```python
from build123d import *

# Parameters (mm, degrees)
ESQUISSE1_R             = 1.75
BOSS_EXTRU_1_DEPTH      = 2
ESQUISSE2_R             = 3
ESQUISSE2_R_2           = 1.5621
ESQUISSE2_R_3           = 1.315256363
BOSS_EXTRU_2_DEPTH      = 4
ENL_V_START             = -4
ESQUISSE4_R             = 1.5621
ESQUISSE4_R_2           = 1.315256363
ENL_V_MAT_EXTRU_1_DEPTH = 4


with BuildPart() as part:
    # Esquisse1 → Boss.-Extru.1 (new body)
    with BuildSketch(Plane(origin=(0, 0, 0), x_dir=(1, 0, 0), z_dir=(0, 1, 0))):
        with BuildLine():
            Line((80, 50.039706632), (74.039706632, 50.039706632))
            ThreePointArc((74.039706632, 50.039706632), (70.476095897, 48.563610735), (69, 45))
            ThreePointArc((69, 45), (65.778174593, 37.221825407), (58, 34))
            Line((58, 34), (-58, 34))
            ThreePointArc((-58, 34), (-65.778174593, 37.221825407), (-69, 45))
            ThreePointArc((-69, 45), (-70.476095897, 48.563610735), (-74.039706632, 50.039706632))
            Line((-74.039706632, 50.039706632), (-80, 50.039706632))
            ThreePointArc((-80, 50.039706632), (-83.563610735, 48.563610735), (-85.039706632, 45))
            Line((-85.039706632, 45), (-85.039706632, -45))
            ThreePointArc((-85.039706632, -45), (-83.563610735, -48.563610735), (-80, -50.039706632))
            Line((-80, -50.039706632), (-74.039706632, -50.039706632))
            ThreePointArc((-74.039706632, -50.039706632), (-70.476095897, -48.563610735), (-69, -45))
            ThreePointArc((-69, -45), (-65.778174593, -37.221825407), (-58, -34))
            Line((-58, -34), (58, -34))
            ThreePointArc((58, -34), (65.778174593, -37.221825407), (69, -45))
            ThreePointArc((69, -45), (70.476095897, -48.563610735), (74.039706632, -50.039706632))
            Line((74.039706632, -50.039706632), (80, -50.039706632))
            ThreePointArc((80, -50.039706632), (83.563610735, -48.563610735), (85.039706632, -45))
            Line((85.039706632, -45), (85.039706632, 45))
            ThreePointArc((85.039706632, 45), (83.563610735, 48.563610735), (80, 50.039706632))
        make_face()
        with Locations(Location((-80, -45, 0), (0, 0, 270))):
            Circle(ESQUISSE1_R, mode=Mode.SUBTRACT)
        with Locations(Location((-80, 45, 0), (0, 0, 270))):
            Circle(ESQUISSE1_R, mode=Mode.SUBTRACT)
        with Locations(Location((80, -45, 0), (0, 0, 270))):
            Circle(ESQUISSE1_R, mode=Mode.SUBTRACT)
        with Locations(Location((80, 45, 0), (0, 0, 270))):
            Circle(ESQUISSE1_R, mode=Mode.SUBTRACT)
    extrude(amount=BOSS_EXTRU_1_DEPTH)

    # Esquisse2 → Boss.-Extru.2 (add)
    # profile 1 of 6: a face of its own
    with BuildSketch(Plane(origin=(0, 2, 0), x_dir=(1, 0, 0), z_dir=(0, 1, 0))):
        with Locations(Location((-14.9479, 19.291507234, 0), (0, 0, 270))):
            Circle(ESQUISSE2_R)
        with Locations(Location((-14.9479, 19.291507234, 0), (0, 0, 270))):
            Circle(ESQUISSE2_R_2, mode=Mode.SUBTRACT)
    # profile 2 of 6: a face of its own
    with BuildSketch(Plane(origin=(0, 2, 0), x_dir=(1, 0, 0), z_dir=(0, 1, 0))):
        with Locations(Location((-14.9479, -8.724692766, 0), (0, 0, 270))):
            Circle(ESQUISSE2_R)
        with Locations(Location((-14.9479, -8.724692766, 0), (0, 0, 270))):
            Circle(ESQUISSE2_R_3, mode=Mode.SUBTRACT)
    # profile 3 of 6: a face of its own
    with BuildSketch(Plane(origin=(0, 2, 0), x_dir=(1, 0, 0), z_dir=(0, 1, 0))):
        with Locations(Location((-38.4556, -24.1662, 0), (0, 0, 270))):
            Circle(ESQUISSE2_R)
        with Locations(Location((-38.4556, -24.1662, 0), (0, 0, 270))):
            Circle(ESQUISSE2_R_2, mode=Mode.SUBTRACT)
    # profile 4 of 6: a face of its own
    with BuildSketch(Plane(origin=(0, 2, 0), x_dir=(1, 0, 0), z_dir=(0, 1, 0))):
        with Locations(Location((36.6776, -24.1662, 0), (0, 0, 270))):
            Circle(ESQUISSE2_R)
        with Locations(Location((36.6776, -24.1662, 0), (0, 0, 270))):
            Circle(ESQUISSE2_R_2, mode=Mode.SUBTRACT)
    # profile 5 of 6: a face of its own
    with BuildSketch(Plane(origin=(0, 2, 0), x_dir=(1, 0, 0), z_dir=(0, 1, 0))):
        with Locations(Location((36.6776, 24.17, 0), (0, 0, 270))):
            Circle(ESQUISSE2_R)
        with Locations(Location((36.6776, 24.17, 0), (0, 0, 270))):
            Circle(ESQUISSE2_R_2, mode=Mode.SUBTRACT)
    # profile 6 of 6: a face of its own
    with BuildSketch(Plane(origin=(0, 2, 0), x_dir=(1, 0, 0), z_dir=(0, 1, 0))):
        with Locations(Location((-45.9486, 24.17, 0), (0, 0, 270))):
            Circle(ESQUISSE2_R)
        with Locations(Location((-45.9486, 24.17, 0), (0, 0, 270))):
            Circle(ESQUISSE2_R_2, mode=Mode.SUBTRACT)
    extrude(amount=BOSS_EXTRU_2_DEPTH)

    # Esquisse4 → Enlèv. mat.-Extru.1 (cut)
    with BuildSketch(Plane(origin=(0, 2, 0), x_dir=(1, 0, 0), z_dir=(0, 1, 0)).offset(ENL_V_START)):
        with Locations(Location((-45.9486, 24.17, 0), (0, 0, 270))):
            Circle(ESQUISSE4_R)
        with Locations(Location((-14.9479, 19.291507234, 0), (0, 0, 270))):
            Circle(ESQUISSE4_R)
        with Locations(Location((36.6776, 24.17, 0), (0, 0, 270))):
            Circle(ESQUISSE4_R)
        with Locations(Location((36.6776, -24.1662, 0), (0, 0, 270))):
            Circle(ESQUISSE4_R)
        with Locations(Location((-14.9479, -8.724692766, 0), (0, 0, 270))):
            Circle(ESQUISSE4_R_2)
        with Locations(Location((-38.4556, -24.1662, 0), (0, 0, 270))):
            Circle(ESQUISSE4_R)
    extrude(amount=ENL_V_MAT_EXTRU_1_DEPTH, mode=Mode.SUBTRACT)


solid = part.part
```
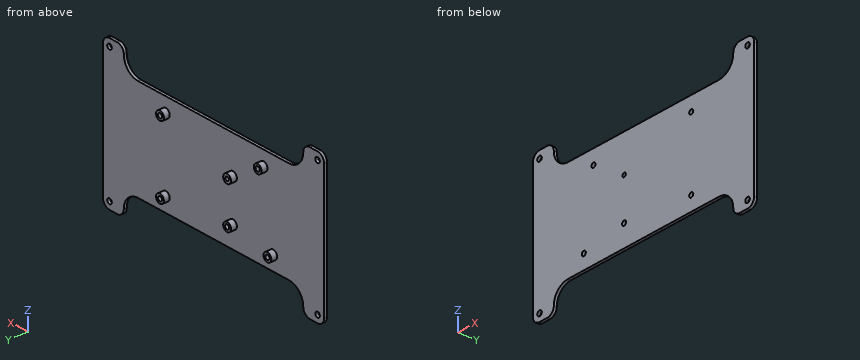
The listing builds one solid part. Answer for the finished solid, in the listing's coordinates (mm). Give positions to 0.01 mm unless a question says otherwise; leave off trailing zeros. Order: outer loops, then holes, each group sorted by start corner. A loop starts at its lowest first (then second) coordinate and runs counter-clockwise, first axis right, second up. Notation, with made-up numbers: (-28, 21.25) -> (25, 21.25) arc R19 ccw to (25, 29.25) -> close; hole circle Ø10 at (86.25, 4). An arc over 180 degrees is marked (long way). One line per item, written item: value.
1) Find section B-B, the plane z = -37. Determine the outline of the cut face in (x, y).
Reported:
outline: (-85.04, 0) -> (-65.55, 0) -> (-65.55, 2) -> (-85.04, 2) -> close; (65.55, 0) -> (85.04, 0) -> (85.04, 2) -> (65.55, 2) -> close
2) Find section D-D, the plane z = -12. Determine the outline of the cut face in (x, y), plus the area to 3 significant figures.
Reported:
outline: (-85.04, 0) -> (85.04, 0) -> (85.04, 2) -> (-85.04, 2) -> close
area: 340 mm^2
3) Flat-ended cylindrical pins translate along their axes: P1, Ø1.6, axis at x = -9, y = 0.5, coming from the +Z side; P2, Ø10, axis at x = -65.5, z = 0.5, coming from the +Y side; P3, Ø1.6, axis at x = 8, y = 1, coming from the -Z side; P4, Ø5, axis at x = -38.46, z = 24.17, coming from the -Y side. Find the tip coordinate at first contact, or state that the pin passes through.
Reported:
P1: stops at z = 34
P2: stops at y = 2
P3: stops at z = -34
P4: stops at y = 0
4) Find section C-C, the plane z = 38. Determine the outline of the cut face in (x, y), plus the area to 3 significant figures.
Reported:
outline: (-85.04, 0) -> (-66.49, 0) -> (-66.49, 2) -> (-85.04, 2) -> close; (66.49, 0) -> (85.04, 0) -> (85.04, 2) -> (66.49, 2) -> close
area: 74.2 mm^2
5) Find the intervals of material crossed by line 1 (X direction, y = 3.5, z = -24.17); line 2 (X direction, y = 1.3, z = 45); line 3 (Z direction, x = -80, y = 0.5), in increasing order.
Reported:
line 1: x = -48.95 to -47.51, -44.39 to -42.95, 33.68 to 35.12, 38.24 to 39.68
line 2: x = -85.04 to -81.75, -78.25 to -69, 69 to 78.25, 81.75 to 85.04
line 3: z = -50.04 to -46.75, -43.25 to 43.25, 46.75 to 50.04
6) Find section A-A, the plane y = 4.5. Count the separate pieces of the cut face and the enclosed holes in it, plus the area to 3 significant figures.
Reported:
separate pieces: 6
enclosed holes: 6
area: 126 mm^2
